Design review of the part built by this model. Coordinates are the model's own, in mm. A direction names the side the tool comes from. Round coordinates to 2 decimals unless told otherwise and drop trailing zeros. Order: outer loops, then holes, each group sorted by start corner. A loop starts at its lowest first (then second) coordinate and runs counter-clockwise, first axis right, second up. Notation, with made-up numbers: M -15,20 L 3,20 A24 ccw 3,32 Z; hole C 54.25,52.25 d9. An arc over 180 degrees is marked long. Use a Markdown table: item, result. Add a question column.
(1) To check wall thickness, follow probe 1 along Y at (x, z) = (0, 1.15); probe 2 along Z at (x, y) = (-3, -6.5); probe 3 along Y at (x, z) = (13.5, 3). State the ranges of each line that lie inside material, in increasing order. Write a range as from..to.
(2) Take a section at D-D (x = 21.5). Write out the cut boundary in (y, z).
(3) Machinability: for faces 4 (the face through (-9.634, 3.034, 0.986)), 5 (the face through (0, -13, 0)), which of the approach directions +Z, -Z, +X, -X, +Y, -Y give a long, thin tool a straight path to every point of the face, cutting with its end or side? Answer none if there is none.
(4) For pin 1 (1 mm diameter, centred on x = -18.5, z = 1.5, fed in from -Y); pin 2 (3 mm diameter, centred on y = 8.5, z = 4, fed in from +X); pin 3 (1 mm diameter, centred on y = -12.5, z = 3.5, fed in from -X), all flat-tipped, find the tip position at first contact; note any pin that passes through.
(5) Take a section at C-C (y = -25.5). Write out the cut boundary in (x, z).
(6) The part is to be moulded in two halves that separate along Y. For faces 1 (the face through (28.14, 8.86, 2.46)), 2 (the face through (0, 0, 2)), 3 (the face through (0, 0, 5)), say which applies: released by +Y, released by -Y, zero draft, split by the parting line, or undercut.
(7) Take a section at A-A (y = 0). Write out the cut boundary in (x, z), then the cut area to 3 significant figures.
(8) Take a section at B-B (x = 1). Write out the cut boundary in (y, z).
```python
from build123d import *

# Parameters (mm, degrees)
SKETCH2_R           = 29.5
BOSS_EXTRUDE1_DEPTH = 60
CUT_REVOLVE1_ANGLE  = 180
CUT_EXTRUDE1_REACH  = 12
SKETCH5_W           = 91.768804765
SKETCH5_H           = 88.75511019
SKETCH6_R           = 10.1
CUT_EXTRUDE2_DEPTH  = 2
SKETCH7_W           = 64.282541495
SKETCH7_H           = 65.701050647
CUT_EXTRUDE3_DEPTH  = 45


with BuildPart() as part:
    # Sketch2 → Boss-Extrude1 (new body)
    with BuildSketch(Plane.XY):
        Circle(SKETCH2_R)
    extrude(amount=BOSS_EXTRUDE1_DEPTH)

    # Sketch4 → Cut-Revolve1 (revolve, cut)
    with BuildSketch(Plane.XY.offset(55)):
        with BuildLine():
            Line((-16.25, 0), (16.25, 0))
            ThreePointArc((16.25, 0), (0, 16.25), (-16.25, 0))
        make_face()
    revolve(axis=Axis((-16.25, 0, 55), (-1, 0, 0)), revolution_arc=CUT_REVOLVE1_ANGLE, mode=Mode.SUBTRACT)

    # Sketch5 → Cut-Extrude1 (cut, up to next)
    with BuildSketch(Plane.XY.offset(50), mode=Mode.PRIVATE) as cut_extrude1_sk1:
        with Locations((1.214417884, -2.093280901)):
            Rectangle(SKETCH5_W, SKETCH5_H)
    cut_extrude1_tool1 = extrude(cut_extrude1_sk1.sketch, amount=CUT_EXTRUDE1_REACH, mode=Mode.PRIVATE) & part.part
    add(cut_extrude1_tool1.solids().sort_by_distance((1.214418, -2.093281, 50))[0], mode=Mode.SUBTRACT)

    # Sketch6 → Cut-Extrude2 (cut)
    with BuildSketch(Plane(origin=(0, 0, 0), x_dir=(-1, 0, 0), z_dir=(0, 0, -1))):
        Circle(SKETCH6_R)
    extrude(amount=-CUT_EXTRUDE2_DEPTH, mode=Mode.SUBTRACT)

    # Sketch7 → Cut-Extrude3 (cut)
    with BuildSketch(Plane.XY.offset(50)):
        with Locations((0.667192443, 0.630931985)):
            Rectangle(SKETCH7_W, SKETCH7_H)
    extrude(amount=-CUT_EXTRUDE3_DEPTH, mode=Mode.SUBTRACT)


solid = part.part
```
Verdict:
| question | item | result |
|---|---|---|
| 1 | probe 1 | y = -29.5..-10.1, 10.1..29.5 |
| 1 | probe 2 | z = 2..5 |
| 1 | probe 3 | y = -26.23..26.23 |
| 2 | outline | M -20.2,0 L 20.2,0 L 20.2,5 L -20.2,5 Z |
| 3 | face 4 | -Z |
| 3 | face 5 | -Z, +X, -X, +Y, -Y |
| 4 | pin 1 | stops at y = -23.37 |
| 4 | pin 2 | stops at x = 28.66 |
| 4 | pin 3 | stops at x = -26.95 |
| 5 | outline | M -14.83,0 L 14.83,0 L 14.83,5 L -14.83,5 Z |
| 6 | face 1 | split by the parting line |
| 6 | face 2 | undercut |
| 6 | face 3 | zero draft |
| 7 | outline | M -29.5,0 L -10.1,0 L -10.1,2 L 10.1,2 L 10.1,0 L 29.5,0 L 29.5,5 L -29.5,5 Z |
| 7 | area | 255 mm^2 |
| 8 | outline | M -29.48,0 L -10.05,0 L -10.05,2 L 10.05,2 L 10.05,0 L 29.48,0 L 29.48,5 L -29.48,5 Z |
